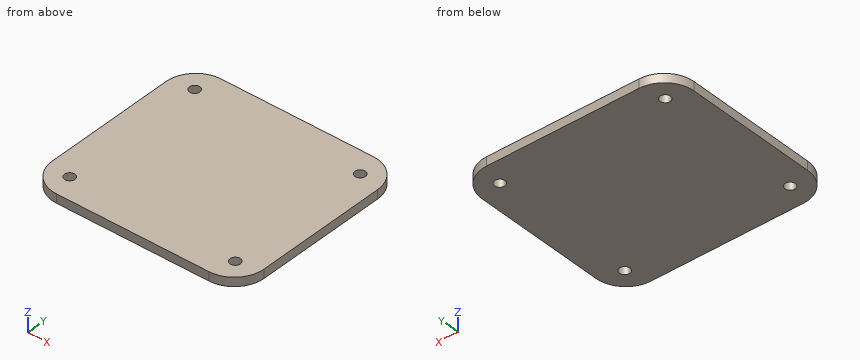
```python
from build123d import *

# Parameters (mm, degrees)
SKETCH_1_W      = 71.296296296
SKETCH_1_H      = 64.814814815
SKETCH_1_R      = 1.75
SKETCH_1_W_2    = 45.37037037
SKETCH_1_H_2    = 38.888888889
EXTRUDE_1_DEPTH = 3
FILLET_1_R      = 10


with BuildPart() as part:
    # 草图1 → 凸台-拉伸1 (new body)
    with BuildSketch(Plane.XY):
        with Locations((0.329915923, 0.017888572)):
            Rectangle(SKETCH_1_W, SKETCH_1_H)
        with Locations((-27.540454447, -24.611741059)):
            Circle(SKETCH_1_R, mode=Mode.SUBTRACT)
        with Locations((28.200286294, -24.611741059)):
            Circle(SKETCH_1_R, mode=Mode.SUBTRACT)
        with Locations((28.200286294, 24.647518201)):
            Circle(SKETCH_1_R, mode=Mode.SUBTRACT)
        with Locations((-27.540454447, 24.647518201)):
            Circle(SKETCH_1_R, mode=Mode.SUBTRACT)
        with Locations((0.329915923, 0.017888572)):
            Rectangle(SKETCH_1_W_2, SKETCH_1_H_2, mode=Mode.SUBTRACT)
        with Locations((0.329915923, 0.017888572)):
            Rectangle(SKETCH_1_W_2, SKETCH_1_H_2)
    extrude(amount=EXTRUDE_1_DEPTH)

    # 圆角1
    fillet_1_edges = [part.edges().sort_by_distance(p)[0] for p in [
        (35.978064071, 32.425295979, 1.5),
        (35.978064071, -32.389518836, 1.5),
        (-35.318232225, -32.389518836, 1.5),
        (-35.318232225, 32.425295979, 1.5),
    ]]
    fillet(fillet_1_edges, radius=FILLET_1_R)


solid = part.part
```
Input: part model. Units: mm. Frame: model coordinates. Give positions to 0.01 mm unless a question says otherwise; leave off trailing zeros. Write each loop counter-clockwise with the first axis right and the second up, starting at its lowest first coordinate (ties: lowest second). Pieces come first, ordered by that corner, then holes. Notation, with made-up numbers: (81.25, 67) - (118.25, 67) arc R29 ccw to (118.25, 90) - close; hole circle Ø8 at (81, 56). An arc over 180 degrees is marked (long way). Write item = value, one per line. Start each with the question number.
1. Ray query, L1, parallel to Y at x = 29, z = 0.8; L2, parallel to X at y = 26, z = 2.1; L3, parallel to X at y = 23.5, z = 1.8. Return the intervals inside material, ascending.
2. First-contact query: pin 1 Ø2 at (x, y) = (28.2, 24.65) entering from -Z. Flat tip, straight axial feed; report the tip coordinate or a pass-through.
3. Section query A-A, the plane z = 2.55. Output: boundary loops of the cut face in (x, y).
Check sheet entries:
q1.L1 = -31.92 to -26.17, -23.06 to 23.09, 26.2 to 31.96
q1.L2 = -34.66 to -28.65, -26.43 to 27.09, 29.31 to 35.32
q1.L3 = -35.26 to -28.86, -26.22 to 26.88, 29.52 to 35.92
q2.pin_1 = through
q3.outline = (-35.32, -22.39) arc R10 ccw to (-25.32, -32.39) - (25.98, -32.39) arc R10 ccw to (35.98, -22.39) - (35.98, 22.43) arc R10 ccw to (25.98, 32.43) - (-25.32, 32.43) arc R10 ccw to (-35.32, 22.43) - close; hole circle Ø3.5 at (-27.54, -24.61); hole circle Ø3.5 at (-27.54, 24.65); hole circle Ø3.5 at (28.2, -24.61); hole circle Ø3.5 at (28.2, 24.65)
